from build123d import *

# Parameters (mm, degrees)
RESSALTO_EXTRUS_O1_DEPTH   = 20
CORTE_EXTRUS_O1_DEPTH      = 35.724775606
CORTE_EXTRUS_O1_DEPTH_BACK = 35.724775606
ESBO_O2_R                  = 1.75
CORTE_EXTRUS_O2_DEPTH      = 3.5
FILETE1_R                  = 1.5
ESBO_O4_W                  = 2.5
ESBO_O4_H                  = 20
RESSALTO_EXTRUS_O2_DEPTH   = 5
ESBO_O5_R                  = 2.25
CORTE_EXTRUS_O3_DEPTH      = 35.749964678
FILETE2_DEPTH              = 7.7499999
FILETE2_START              = 12.2500001
FILETE2_2_DEPTH            = 7.7499999
FILETE2_START_2            = 7.7499999
FILETE2_3_DEPTH            = 4.5000002
FILETE2_START_3            = -2.9
FILETE2_4_OUTLINE_R        = 2.25
FILETE2_4_DEPTH            = 7.998725805
ESBO_O6_R                  = 5.5
CORTE_EXTRUS_O4_DEPTH      = 10


with BuildPart() as part:
    # Esboço1 → Ressalto-extrusão1 (new body)
    with BuildSketch(Plane.XY):
        with BuildLine():
            ThreePointArc((10.599999813, 0.1), (11.660659985, -0.339339828), (12.099999813, -1.4))
            Line((12.099999813, -1.4), (12.099999813, -2.9))
            Line((12.099999813, -2.9), (24.100000848, -2.9))
            Line((24.100000848, -2.9), (24.100000848, -7.9))
            Line((24.100000848, -7.9), (-20.099999152, -7.9))
            Line((-20.099999152, -7.9), (-20.099999152, -2.9))
            Line((-20.099999152, -2.9), (-8.099998116, -2.9))
            Line((-8.099998116, -2.9), (-8.099998116, 2.1))
            ThreePointArc((-8.099998116, 2.1), (-6.635532022, 5.635533906), (-3.099998116, 7.1))
            Line((-3.099998116, 7.1), (12.099999813, 7.1))
            Line((12.099999813, 7.1), (12.099999813, 2.6))
            ThreePointArc((12.099999813, 2.6), (11.660659985, 1.539339828), (10.599999813, 1.1))
            Line((10.599999813, 1.1), (3.949683532, 1.1))
            ThreePointArc((3.949683532, 1.1), (-4.055174785, -0.604613482), (4.098780306, 0.1))
            Line((4.098780306, 0.1), (10.599999813, 0.1))
        make_face()
    extrude(amount=RESSALTO_EXTRUS_O1_DEPTH)

    # Esboço2 → Corte-extrusão1 (cut, two sides: drawn at the far end of the back side and taken through both)
    with BuildSketch(Plane(origin=(0, 7.1, 0), x_dir=(1, 0, 0), z_dir=(0, 1, 0)).offset(-CORTE_EXTRUS_O1_DEPTH_BACK)):
        with Locations(Location((8.400001366, -10, 0), (0, 0, 180))):
            Circle(ESBO_O2_R)
    extrude(amount=CORTE_EXTRUS_O1_DEPTH + CORTE_EXTRUS_O1_DEPTH_BACK, mode=Mode.SUBTRACT)

    # Esboço3 → Corte-extrusão2 (cut)
    with BuildSketch(Plane.XZ.offset(7.9)):
        Polygon((8.400001366, 13.348631561), (5.500001366, 11.674315781), (5.500001366, 8.325684219), (8.400001366, 6.651368439), (11.300001366, 8.325684219), (11.300001366, 11.674315781), align=None)
    extrude(amount=-CORTE_EXTRUS_O2_DEPTH, mode=Mode.SUBTRACT)

    # Filete1
    filete1_edges = [part.edges().sort_by_distance(p)[0] for p in [
        (12.099999813, -2.9, 10),
    ]]
    fillet(filete1_edges, radius=FILETE1_R - 0.0001)  # a hair under: the kernel refuses the full size

    # Esboço4 → Ressalto-extrusão2 (add)
    with BuildSketch(Plane.XZ.offset(7.9)):
        with Locations((-21.349999152, 10)):
            Rectangle(ESBO_O4_W, ESBO_O4_H)
        with Locations((25.350000848, 10)):
            Rectangle(ESBO_O4_W, ESBO_O4_H)
    extrude(amount=-RESSALTO_EXTRUS_O2_DEPTH)

    # Esboço5 → Corte-extrusão3 (cut, through all)
    with BuildSketch(Plane(origin=(0, -2.9, 0), x_dir=(1, 0, 0), z_dir=(0, 1, 0))):
        with Locations(Location((-15.349998634, -10, 0), (0, 0, 180))):
            Circle(ESBO_O5_R)
        with Locations(Location((20.100000331, -10, 0), (0, 0, 180))):
            Circle(ESBO_O5_R)
    extrude(amount=-CORTE_EXTRUS_O3_DEPTH, mode=Mode.SUBTRACT)

    # Filete2: read off the stored shape, not the designer's step
    # Filete2 outline → Filete2 (add)
    with BuildSketch(Plane.XY):
        with BuildLine():
            ThreePointArc((-7.100953445, 5.098725805), (-13.932624155, -0.679149409), (-22.599999152, -2.9))
            Line((-22.599999152, -2.9), (-8.099998116, -2.9))
            Line((-8.099998116, -2.9), (-8.099998116, 2.1))
            ThreePointArc((-8.099998116, 2.1), (-7.843666351, 3.680383396), (-7.100953445, 5.098725805))
        make_face()
    extrude(amount=FILETE2_DEPTH)

    # Filete2 2 outline → Filete2 2 (add)
    with BuildSketch(Plane.XY.offset(FILETE2_START)):
        with BuildLine():
            ThreePointArc((-7.100953445, 5.098725805), (-13.932624155, -0.679149409), (-22.599999152, -2.9))
            Line((-22.599999152, -2.9), (-8.099998116, -2.9))
            Line((-8.099998116, -2.9), (-8.099998116, 2.1))
            ThreePointArc((-8.099998116, 2.1), (-7.843666351, 3.680383396), (-7.100953445, 5.098725805))
        make_face()
    extrude(amount=FILETE2_2_DEPTH)

    # Filete2 3 outline → Filete2 3 (add)
    with BuildSketch(Plane.XY.offset(FILETE2_START_2)):
        with BuildLine():
            ThreePointArc((-7.100953445, 5.098725805), (-13.932624155, -0.679149409), (-22.599999152, -2.9))
            Line((-22.599999152, -2.9), (-8.099998116, -2.9))
            Line((-8.099998116, -2.9), (-8.099998116, 2.099999998))
            ThreePointArc((-8.099998116, 2.099999998), (-7.843666351, 3.680383395), (-7.100953445, 5.098725805))
        make_face()
    extrude(amount=FILETE2_3_DEPTH)

    # Filete2 4 outline → Filete2 4 (cut)
    with BuildSketch(Plane(origin=(0, 0, 0), x_dir=(1, 0, 0), z_dir=(0, 1, 0)).offset(FILETE2_START_3)):
        with Locations((-15.349998634, -10)):
            Circle(FILETE2_4_OUTLINE_R)
    extrude(amount=FILETE2_4_DEPTH, mode=Mode.SUBTRACT)

    # Esboço6 → Corte-extrusão4 (cut)
    with BuildSketch(Plane(origin=(0, 7.1, 0), x_dir=(1, 0, 0), z_dir=(0, 1, 0))):
        with Locations(Location((-15.349998634, -10, 0), (0, 0, 180))):
            Circle(ESBO_O6_R)
    extrude(amount=-CORTE_EXTRUS_O4_DEPTH, mode=Mode.SUBTRACT)


solid = part.part
Read the model definition and answer for the solid it produces. Units are mm, in the model's axes. A direction names the side the tool comes from. Coordinates: 2 decimals unless noted, no trailing zeros. Loops run counter-clockwise (first coordinate to the right, second up) from the corner with the lowest first, then second, coordinate; pieces in that order, holes last. Notation, with made-up numbers: (-23.75, 84.25) -> (29.25, 84.25) arc R37 ccw to (29.25, 122.25) -> close; hole circle Ø11 at (-24.75, 18.5). An arc over 180 degrees is marked (long way). Write item = value, one per line. Start each with the question number.
1) Find the intervals of material crossed by L1, parallel to Y at x = 6, z = 8; L2, parallel to X at y = 3.25, z = 14; L3, parallel to Y at x = 11.5, z = 19.25, in increasing order. Write a range as from..to.
2) The part is cut by section A-A, the plane x = 0. Determine the outline of the cut face in (y, z).
3) Given P1, Ø6, axis at y = 1, z = 10.5, coming from the +X side; P2, Ø4, axis at x = 21, z = 12, coming from the +Y side; P3, Ø5.5, axis at x = 8.4, z = 10, coming from the +Y side; P4, Ø2, axis at y = 5, z = 8.5, coming from the +X side, each flat-ended and moving along its own axis, determine where each tip first touches the part or whether it passes through.
4) The mould has two halves that part along Z. Classify faces 4 (the face through (12.1, 5, 10)), 5 (the face through (2, -5, 20)), 6 (the face through (9.83, -6.174, 7.477)), 7 (the face through (2, -5, 0)): pulls with the +Z half, pulls with the -Z half, needs draft (parallel to the pull), parting line crosses it, or undercut.
5) The part is cut by section D-D, the plane y = -5.25. Determine the outline of the cut face in (x, z), plus the area to 3 significant figures.
6) For faces 1 (the face through (11.65, -0.33, 9.86)), 2 (the face through (5.5, -6, 10)), 3 (the face through (20, -2.9, 7.6)), determine the directions among +Z, -Z, +X, -X, +Y, -Y from which every point of the face is accessible in a straight line to the end or side of a thin tool.
7) The part is cut by section B-B, the plane y = -2.25. Determine the outline of the cut face in (x, z).
Result:
q1.L1 = -7.9..0.1, 1.1..7.1
q1.L2 = -8.67..-2.5, 2.5..12.1
q1.L3 = -7.9..-0.2, 1.4..7.1
q2.outline = (-7.9, 0) -> (-4.1, 0) -> (-4.1, 20) -> (-7.9, 20) -> close; (4.1, 0) -> (7.1, 0) -> (7.1, 20) -> (4.1, 20) -> close
q3.P1 = 12.23
q3.P2 = -2.9
q3.P3 = 7.1
q3.P4 = 12.1
q4.face_4 = needs draft
q4.face_5 = pulls with the +Z half
q4.face_6 = undercut
q4.face_7 = pulls with the -Z half
q5.outline = (-22.6, 0) -> (26.6, 0) -> (26.6, 20) -> (-22.6, 20) -> close; hole circle Ø4.5 at (-15.35, 10); hole (5.5, 8.33) -> (8.4, 6.65) -> (11.3, 8.33) -> (11.3, 11.67) -> (8.4, 13.35) -> (5.5, 11.67) -> close; hole circle Ø4.5 at (20.1, 10)
q5.area = 923 mm²
q6.face_1 = +Z, -Z, +X
q6.face_2 = -Y
q6.face_3 = +Z, -Z, +X, +Y
q7.outline = (-18.02, 0) -> (-3.43, 0) -> (-3.43, 20) -> (-18.02, 20) -> (-18.02, 14.81) arc R5.5 cw (long way) to (-18.02, 5.19) -> close; (3.43, 0) -> (12.36, 0) -> (12.36, 20) -> (3.43, 20) -> close; hole circle Ø3.5 at (8.4, 10)
